Can you work these out from the drawing? Everything is in mm from the part's minimum corner. A direction names the side the tool comes from. Give positions to 0.01 mm unless a question says otherwise; leave off trailing zeros. Order: outer loops, then holes, each group sorted by start corner. A loop starts at its lowest first (then second) coordinate and runs counter-clockwise, first axis right, second up. Notation, with made-up numbers: (-20.75, -30.5) -> (17.25, -30.5) arc R28 cw to (17.25, -10.5) -> close; hole circle Ø4 at (52, 70.25). An arc over 180 degrees is marked (long way). Answer as CSV lines item,"result". Start each with the question number.
(1) I need wall thicknesses on L1, parallel to Y at x = 48, z = 10; L2, parallel to X at y = 2.3, z = 10; L3, parallel to Z at x = 10, y = 2. Which ranges of each line are inside material? Lowest first, please.
(2) I want a section at C-C (x = 10). Please give me the cut outline in (y, z), plus the area to 3 significant figures.
(3) I want a section at A-A (y = 6). Please give me the cut outline in (x, z), plus the area to 3 significant figures.
(4) I want a section at D-D (z = 7.25). Please give me the cut outline in (x, y).
(5) We'd pull the mould along X, two halves only. Please class the marked faces 1, 2 and 3: released by +X, released by -X, zero draft, split by the parting line, or undercut.
(6) Will these pins go through, and if not, where does the flat tip stop? pin 1 Ø6 at (y, z) = (13.5, 13.5) entering from -X; pin 2 Ø6 at (y, z) = (12, 8) entering from +X; pin 3 Ø5 at (y, z) = (18, 10) entering from -X.
(7) I want a section at B-B (y = 18). Please give me the cut outline in (x, z).
(8) On a 3-axis mill with a long thin cutter (end or side, diameter ignored), from which of +Z, -Z, +X, -X, +Y, -Y can I reach the whole of each face in a straight line? I mean the marked faces 4, 5, 6, 7 and 8. Say none if no direction works.
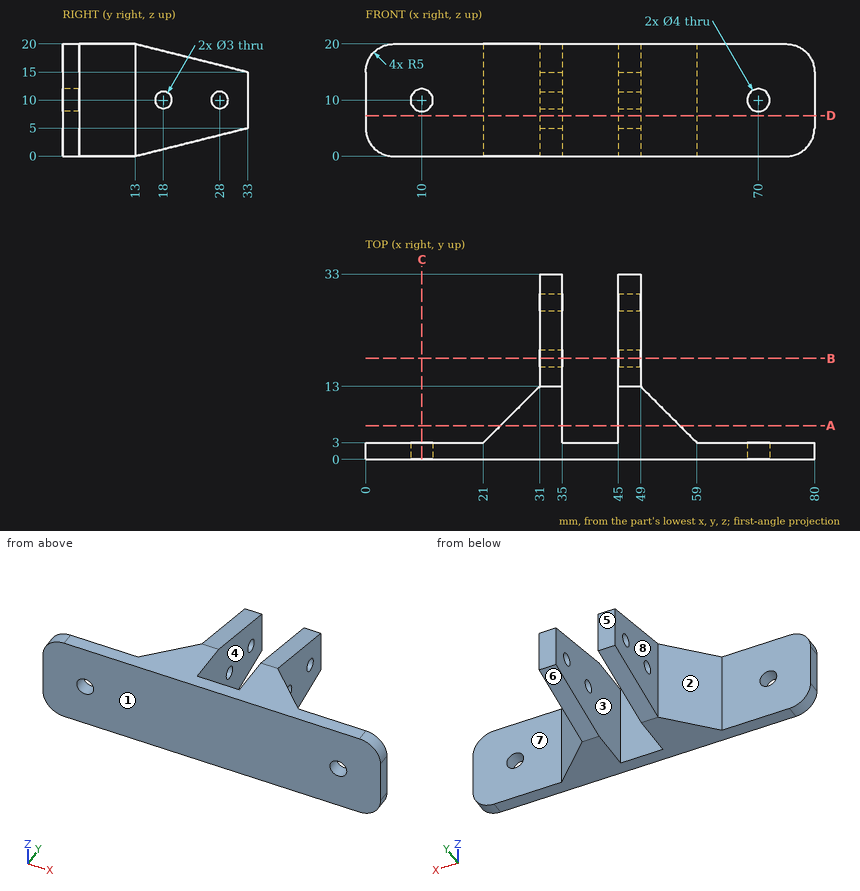
Final values:
1,L1,"0 to 16.5, 19.5 to 26.5, 29.5 to 33"
1,L2,"0 to 8, 12 to 68, 72 to 80"
1,L3,"0 to 8, 12 to 20"
2,outline,"(0, 0) -> (3, 0) -> (3, 8) -> (0, 8) -> close; (0, 12) -> (3, 12) -> (3, 20) -> (0, 20) -> close"
2,area,"48.0 mm²"
3,outline,"(24, 0) -> (35, 0) -> (35, 20) -> (24, 20) -> close; (45, 0) -> (56, 0) -> (56, 20) -> (45, 20) -> close"
3,area,"440 mm²"
4,outline,"(0, 0) -> (80, 0) -> (80, 3) -> (59, 3) -> (49, 13) -> (49, 33) -> (45, 33) -> (45, 3) -> (35, 3) -> (35, 33) -> (31, 33) -> (31, 13) -> (21, 3) -> (0, 3) -> close"
5,face 1,"zero draft"
5,face 2,"released by -X"
5,face 3,"undercut"
6,pin 1,"x = 28.5"
6,pin 2,"x = 53"
6,pin 3,"x = 31"
7,outline,"(31, 1.25) -> (35, 1.25) -> (35, 8.5) -> (31, 8.5) -> close; (31, 11.5) -> (35, 11.5) -> (35, 18.75) -> (31, 18.75) -> close; (45, 1.25) -> (49, 1.25) -> (49, 8.5) -> (45, 8.5) -> close; (45, 11.5) -> (49, 11.5) -> (49, 18.75) -> (45, 18.75) -> close"
8,face 4,"+Z, -Z, +Y"
8,face 5,"+Z, -Z, +X, -X, +Y"
8,face 6,"-Z, +X, -X, +Y"
8,face 7,"+Z, -Z, +X, +Y"
8,face 8,"+Z, -Z, -X, +Y"
